Design review of the part built by this model. Coordinates are the model's own, in mm. Face numbers are marked on the shaded views. Coordinates: 2 decimals unless noted, no trailing zeros. Write each loop counter-clockwise with the first axis right and the second up, starting at its lowest first coordinate (ties: lowest second). Pieces come first, ordered by that corner, then holes.
Q1. Take a section at D-D, the plane z = -3. Write out the cut boundary in (x, y).
Q2. Take a section at C-C, the plane x = 17. Write out the cut boundary in (y, z), plus the area to 3 significant figures.
Q3. For L1, parallel to Y at x = 3.5, z = 0; L2, parallel to Y at x = 0.6, z = 0; L3, parallel to X at y = -1, z = 3.25, list the stretches that pass through material, from the lowest coordinate up.
Q4. Take a section at A-A, the plane y = 0. Write out the cut boundary in (x, z), plus the area to 3 significant figures.
Q5. The part is to be moulded in two halves that separate along Z. For the marked faces 1, 2 and 3, say which applies: released by +Z, released by -Z, zero draft, split by the parting line, or undercut.
Q6. For pin 1 Ø3.5 at (y, z) = (-0.5, -1) entering from +X; pin 2 Ø1 at (y, z) = (0.5, -0.5) entering from -X; pin 3 Ø1 at (y, z) = (-4.5, -2.5) entering from -X; pin 4 Ø4 at (x, y) = (16.5, -4) entering from +Z, all flat-tipped, find the tip position at first contact; note any pin that passes through.
from build123d import *


with BuildPart() as part:
    # Esboço1 → Revolução1 (revolve)
    with BuildSketch(Plane(origin=(0, 0, 0), x_dir=(1, 0, 0), z_dir=(0, 1, 0)), mode=Mode.PRIVATE) as revolu_o1_sk:
        Polygon((3.8, 1.05), (2.960398706, 1.05), (2.960398706, 2.25), (0, 2.25), (0, 5.55), (1.4, 5.55), (1.4, 4.8), (33, 4.8), (33, 4.5), (3.8, 4.5), align=None)
    revolve(revolu_o1_sk.sketch.rotate(Axis((0, 0, 0), (1, 0, 0)), 180), axis=Axis((0, 0, 0), (1, 0, 0)))


solid = part.part
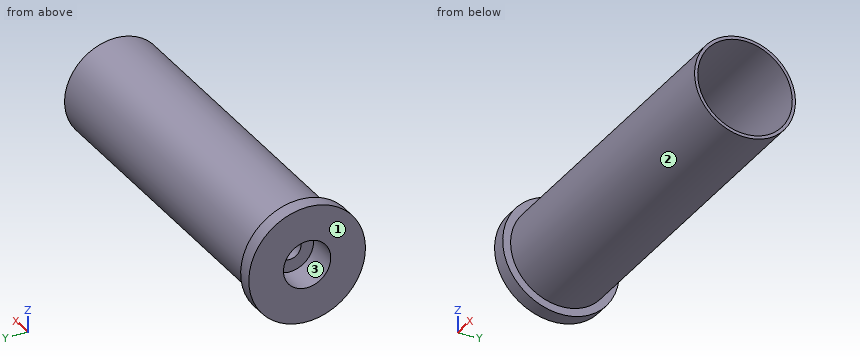
Responses:
1. outline: (0, -4.67) - (1.4, -4.67) - (1.4, -3.75) - (33, -3.75) - (33, -3.35) - (3.8, -3.35) - (3.8, 3.35) - (33, 3.35) - (33, 3.75) - (1.4, 3.75) - (1.4, 4.67) - (0, 4.67) - close
2. outline: circle Ø9.6 at (0, 0); hole circle Ø9 at (0, 0)
2. area: 8.77 mm2
3. L1: y = -4.8 to -1.05, 1.05 to 4.8
3. L2: y = -5.55 to -2.25, 2.25 to 5.55
3. L3: x = 0 to 3.8
4. outline: (0, -5.55) - (1.4, -5.55) - (1.4, -4.8) - (33, -4.8) - (33, -4.5) - (3.8, -4.5) - (3.8, -1.05) - (2.96, -1.05) - (2.96, -2.25) - (0, -2.25) - close; (0, 2.25) - (2.96, 2.25) - (2.96, 1.05) - (3.8, 1.05) - (3.8, 4.5) - (33, 4.5) - (33, 4.8) - (1.4, 4.8) - (1.4, 5.55) - (0, 5.55) - close
4. area: 41.0 mm2
5. face 1: zero draft
5. face 2: split by the parting line
5. face 3: undercut
6. pin 1: stops at x = 3.8
6. pin 2: stops at x = 2.96
6. pin 3: stops at x = 0
6. pin 4: stops at z = 4.36
